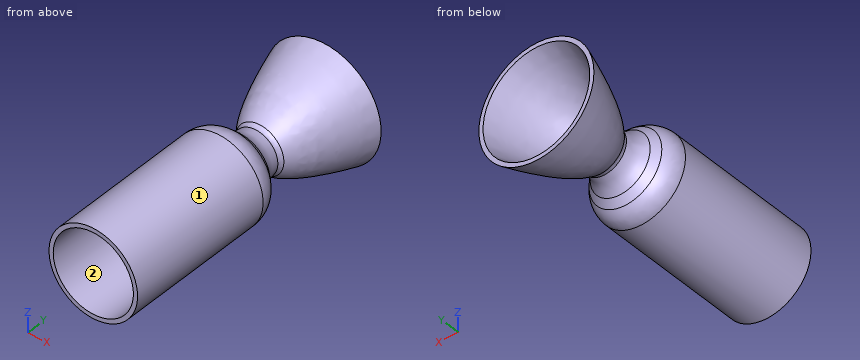
```python
from build123d import *


with BuildPart() as part:
    # Sketch1 → Revolve2 (revolve)
    with BuildSketch(Plane.XY, mode=Mode.PRIVATE) as revolve2_sk:
        with BuildLine():
            Line((71.727523603, 109.92750764), (77.388416165, 109.92750764))
            add(Edge.make_bspline(
                [(32.495712479, 6.492229985), (54.951080007, 34.627531396), (77.388416165, 109.92750764)],
                knots=[0, 0, 0, 1, 1, 1], degree=2))
            add(Edge.make_bspline(
                [(29.79950115, -0.017009666), (29.799501776, 0.018882986), (29.800039607, 0.093104024), (29.802456999, 0.250631404), (29.808894844, 0.410054451), (29.820966875, 0.629754601), (29.841868363, 0.884423662), (29.875617995, 1.185527607), (29.926932581, 1.525040832), (29.990976977, 1.863987111), (30.067574877, 2.199344754), (30.156756847, 2.532229755), (30.258174689, 2.861082979), (30.372052346, 3.186337375), (30.497630047, 3.506617491), (30.635719253, 3.822657067), (30.784503576, 4.132272519), (30.946445498, 4.437773457), (31.11692178, 4.73429191), (31.302947997, 5.028694196), (31.492221546, 5.30850927), (31.70483875, 5.593717877), (31.87930965, 5.815903982), (32.066779032, 6.032941971), (32.204988524, 6.19163198), (32.370875346, 6.365112113), (32.444953537, 6.441469176), (32.495712479, 6.492229985)],
                knots=[0.082568816, 0.082568816, 0.082568816, 0.082568816, 0.082568816, 0.102426634, 0.122284453, 0.142142271, 0.162000089, 0.201715725, 0.241431362, 0.281146998, 0.320862634, 0.360578271, 0.400293907, 0.440009544, 0.47972518, 0.519440816, 0.559156453, 0.598872089, 0.638587725, 0.678303362, 0.718018998, 0.757734635, 0.797450271, 0.837165907, 0.857023726, 0.876881544, 0.91659718, 0.91659718, 0.91659718, 0.91659718, 0.91659718], degree=4))
            add(Edge.make_bspline(
                [(29.79950115, -0.017009666), (29.799502381, -0.087538311), (29.800031528, -0.230593853), (29.802407213, -0.56019258), (29.808731607, -0.84117006), (29.818216728, -1.211831735), (29.830859021, -1.530444722), (29.846659245, -1.878949267), (29.865614504, -2.210716535), (29.893252118, -2.635079064), (29.932720324, -3.139043611), (30.003732985, -3.896988339), (30.123559956, -4.903460052), (30.299919323, -6.073720425), (30.551318512, -7.40217608), (30.852228593, -8.72058418), (31.202203904, -10.026646875), (31.600794265, -11.318829264), (32.047378674, -12.595109003), (32.541436606, -13.853897152), (33.082106405, -15.093206798), (33.668912671, -16.311619464), (34.300572682, -17.506948466), (34.976965681, -18.67829743), (35.695878388, -19.822753071), (36.458455286, -20.94086975), (37.15960048, -21.891421437), (37.789169411, -22.690455158), (38.324561704, -23.337431817), (38.772689056, -23.857014696), (39.208883315, -24.346825927), (39.63625941, -24.805494071), (39.945991929, -25.130877992), (40.237293247, -25.426658729), (40.336845715, -25.526959614), (40.386716092, -25.5768318)],
                knots=[0.082637729, 0.082637729, 0.082637729, 0.082637729, 0.082637729, 0.092574926, 0.102512123, 0.11244932, 0.122386517, 0.132323714, 0.142260911, 0.152198108, 0.162135305, 0.182009699, 0.201884093, 0.24163288, 0.281381668, 0.321130456, 0.360879243, 0.400628031, 0.440376819, 0.480125606, 0.519874394, 0.559623181, 0.599371969, 0.639120757, 0.678869544, 0.718618332, 0.75836712, 0.798115907, 0.817990301, 0.837864695, 0.857739089, 0.877613483, 0.897487877, 0.907425074, 0.91736227, 0.91736227, 0.91736227, 0.91736227, 0.91736227], degree=4))
            Line((40.386716092, -25.5768318), (48.994344291, -34.184459998))
            add(Edge.make_bspline(
                [(59.581960968, -59.744683548), (59.581959736, -59.674153485), (59.581430593, -59.532576432), (59.579054743, -59.198734945), (59.572730144, -58.921965822), (59.563244656, -58.549737817), (59.550601759, -58.230007951), (59.530850931, -57.798764772), (59.500838589, -57.298130228), (59.456626426, -56.705168494), (59.377721756, -55.865650695), (59.277860165, -55.025336189), (59.157109089, -54.189605759), (58.987244125, -53.189595569), (58.792497489, -52.194613151), (58.566808422, -51.205709413), (58.310447525, -50.224659368), (58.029722641, -49.25024807), (57.724782039, -48.283139554), (57.33397113, -47.166305397), (56.839953659, -45.907578736), (56.29916705, -44.668139134), (55.712494225, -43.449871857), (55.080553527, -42.25426357), (54.404558525, -41.083325211), (53.684908815, -39.938142989), (52.923535432, -38.821246572), (52.220302354, -37.868622118), (51.593971231, -37.072842456), (51.053250974, -36.420551616), (50.615560241, -35.911417966), (50.215209482, -35.464162991), (49.881890795, -35.101801519), (49.574357917, -34.777510486), (49.374505699, -34.568719785), (49.144825365, -34.335686622), (49.044216443, -34.23433239), (48.994344291, -34.184459998)],
                knots=[0.082637729, 0.082637729, 0.082637729, 0.082637729, 0.082637729, 0.092574926, 0.102512123, 0.11244932, 0.122386517, 0.132323714, 0.142260911, 0.162135305, 0.182009699, 0.201884093, 0.24163288, 0.261507274, 0.281381668, 0.321130456, 0.360879243, 0.380753637, 0.400628031, 0.440376819, 0.480125606, 0.519874394, 0.559623181, 0.599371969, 0.639120757, 0.678869544, 0.718618332, 0.75836712, 0.798115907, 0.817990301, 0.837864695, 0.857739089, 0.877613483, 0.88755068, 0.897487877, 0.907425074, 0.91736227, 0.91736227, 0.91736227, 0.91736227, 0.91736227], degree=4))
            Line((59.581960968, -59.744683548), (59.581960968, -262.944683548))
            Line((59.581960968, -262.944683548), (53.881527661, -262.927513222))
            Line((53.881527661, -262.927513222), (53.881527661, -59.727513222))
            add(Edge.make_bspline(
                [(53.881527661, -59.727513222), (53.88152643, -59.65698316), (53.880997287, -59.515406106), (53.878621437, -59.18156462), (53.872296838, -58.904795496), (53.862811351, -58.532567491), (53.850168454, -58.212837625), (53.830417626, -57.781594446), (53.800405285, -57.280959903), (53.756193122, -56.687998169), (53.677288452, -55.848480369), (53.577426862, -55.008165864), (53.456675787, -54.172435434), (53.286810823, -53.172425243), (53.092064188, -52.177442825), (52.866375121, -51.188539087), (52.610014225, -50.207489042), (52.329289341, -49.233077744), (52.02434874, -48.265969227), (51.633537832, -47.14913507), (51.139520362, -45.890408409), (50.598733754, -44.650968807), (50.012060929, -43.432701529), (49.380120232, -42.237093242), (48.70412523, -41.066154882), (47.984475521, -39.92097266), (47.22310214, -38.804076242), (46.519869062, -37.851451788), (45.893537939, -37.055672125), (45.352817683, -36.403381285), (44.91512695, -35.894247635), (44.514776192, -35.44699266), (44.181457505, -35.084631188), (43.873924626, -34.760340154), (43.674072409, -34.551549453), (43.444392075, -34.31851629), (43.343783154, -34.217162058), (43.293911001, -34.167289665)],
                knots=[0.082637729, 0.082637729, 0.082637729, 0.082637729, 0.082637729, 0.092574926, 0.102512123, 0.11244932, 0.122386517, 0.132323714, 0.142260911, 0.162135305, 0.182009699, 0.201884093, 0.24163288, 0.261507274, 0.281381668, 0.321130456, 0.360879243, 0.380753637, 0.400628031, 0.440376819, 0.480125606, 0.519874394, 0.559623181, 0.599371969, 0.639120757, 0.678869544, 0.718618332, 0.75836712, 0.798115907, 0.817990301, 0.837864695, 0.857739089, 0.877613483, 0.88755068, 0.897487877, 0.907425074, 0.91736227, 0.91736227, 0.91736227, 0.91736227, 0.91736227], degree=4))
            Line((43.293911001, -34.167289665), (34.686282803, -25.559661467))
            add(Edge.make_bspline(
                [(24.099067874, 0.000160672), (24.099069105, -0.070367973), (24.099598252, -0.213423515), (24.101973937, -0.543022242), (24.108298331, -0.823999722), (24.117783452, -1.194661397), (24.130425744, -1.513274384), (24.146225968, -1.861778929), (24.165181227, -2.193546197), (24.19281884, -2.617908726), (24.232287047, -3.121873273), (24.303299707, -3.879818001), (24.423126678, -4.886289715), (24.599486043, -6.056550087), (24.850885233, -7.385005742), (25.151795313, -8.703413843), (25.501770623, -10.009476538), (25.900360983, -11.301658927), (26.346945391, -12.577938666), (26.841003322, -13.836726816), (27.381673121, -15.076036462), (27.968479386, -16.294449128), (28.600139397, -17.48977813), (29.276532395, -18.661127095), (29.995445101, -19.805582736), (30.758021999, -20.923699416), (31.459167192, -21.874251103), (32.088736122, -22.673284825), (32.624128416, -23.320261484), (33.072255767, -23.839844363), (33.508450026, -24.329655594), (33.935826121, -24.788323738), (34.245558639, -25.113707659), (34.536859957, -25.409488397), (34.636412425, -25.509789282), (34.686282803, -25.559661467)],
                knots=[0.082637729, 0.082637729, 0.082637729, 0.082637729, 0.082637729, 0.092574926, 0.102512123, 0.11244932, 0.122386517, 0.132323714, 0.142260911, 0.152198108, 0.162135305, 0.182009699, 0.201884093, 0.24163288, 0.281381668, 0.321130456, 0.360879243, 0.400628031, 0.440376819, 0.480125606, 0.519874394, 0.559623181, 0.599371969, 0.639120757, 0.678869544, 0.718618332, 0.75836712, 0.798115907, 0.817990301, 0.837864695, 0.857739089, 0.877613483, 0.897487877, 0.907425074, 0.91736227, 0.91736227, 0.91736227, 0.91736227, 0.91736227], degree=4))
            add(Edge.make_bspline(
                [(24.099067874, 0.000160672), (24.0990685, 0.036053324), (24.099606331, 0.110274362), (24.102023723, 0.267801742), (24.108461568, 0.427224789), (24.120533599, 0.646924939), (24.141435087, 0.901594), (24.175184719, 1.202697945), (24.226499305, 1.54221117), (24.290543701, 1.881157449), (24.367141601, 2.216515092), (24.456323571, 2.549400093), (24.557741413, 2.878253317), (24.671619071, 3.203507713), (24.797196771, 3.523787829), (24.935285977, 3.839827405), (25.084070301, 4.149442857), (25.246012222, 4.454943795), (25.416488505, 4.751462248), (25.602514721, 5.045864533), (25.79178827, 5.325679608), (26.004405474, 5.610888215), (26.178876374, 5.83307432), (26.366345756, 6.050112309), (26.504555248, 6.208802318), (26.67044207, 6.382282451), (26.744520261, 6.458639514), (26.795279203, 6.509400323)],
                knots=[0.082568816, 0.082568816, 0.082568816, 0.082568816, 0.082568816, 0.102426634, 0.122284453, 0.142142271, 0.162000089, 0.201715725, 0.241431362, 0.281146998, 0.320862634, 0.360578271, 0.400293907, 0.440009544, 0.47972518, 0.519440816, 0.559156453, 0.598872089, 0.638587725, 0.678303362, 0.718018998, 0.757734635, 0.797450271, 0.837165907, 0.857023726, 0.876881544, 0.91659718, 0.91659718, 0.91659718, 0.91659718, 0.91659718], degree=4))
            add(Edge.make_bspline(
                [(26.795279203, 6.509400323), (49.261401403, 34.636114842), (71.727523603, 109.92750764)],
                knots=[0, 0, 0, 1, 1, 1], degree=2))
        make_face()
    revolve(revolve2_sk.sketch.rotate(Axis((-0.005532126, 165.815985114, 0), (0, -1, 0)), 180), axis=Axis((-0.005532126, 165.815985114, 0), (0, -1, 0)))


solid = part.part
```
Can you work these out from the model? Positions are in its coordinate system, mm. Face numbers are marked on the shaded views. Give positions to 0.01 mm unless a question says otherwise; leave off trailing zeros. Write each loop counter-clockwise with the first axis right and the second up, starting at its lowest first coordinate (ties: lowest second). Pieces come first, ordered by that corner, then holes. Notation, with made-up numbers: (87.25, -27.75) - (145.25, -27.75) arc R28 ccw to (145.25, -1.75) - close; hole circle Ø8 at (45.25, -34.5). An arc over 180 degrees is marked (long way). Write item = value, one per line. Start each with the question number.
1. Imagine slicing it at A-A (y = -66.5). Please give me the cut outline in (x, z), and give its area (3 significant figures).
2. For pin 1 (12 mm diameter, centred on x = -11.5, z = -22, fed in from -Y); pin 2 (2 mm diameter, centred on y = 42.5, z = -12.5, fed in from -X); pin 3 (5 mm diameter, centred on y = -191, z = -15, fed in from -X), each with a flat end and sliding along its axis, tell me the tip position at first contact or that it passes through.
3. Please list where these lines run through material, in increasing order: line 1 (X direction, y = -222.5, z = -1); line 2 (Z direction, x = -4.5, y = 32); line 3 (X direction, y = -167, z = -24.5).
4. Thinking about a two-plate mould opening in Z: for the marked faces 1 and 2, which applies, released by +Z, released by -Z, zero draft, split by the parting line, or undercut?
Worked answers:
q1.outline = circle Ø119.17 at (-0.01, 0); hole circle Ø107.77 at (-0.01, 0)
q1.area = 2,030 mm2
q2.pin_1 = -20.99
q2.pin_2 = -52.25
q2.pin_3 = -58.27
q3.line_1 = -59.58 to -53.88, 53.87 to 59.57
q3.line_2 = -48.03 to -42.3, 42.3 to 48.03
q3.line_3 = -54.32 to -48, 47.99 to 54.31
q4.face_1 = split by the parting line
q4.face_2 = undercut
